Model file for the job. Use its own axes, mm. Face numbers are marked on the shaded views. A direction names the side the tool comes from. Round coordinates to 2 decimals unless told otherwise and drop trailing zeros. Loops run counter-clockwise (first coordinate to the right, second up) from the corner with the lowest first, then second, coordinate; pieces in that order, holes last. Notation, with made-up numbers: (64, 49.5) -> (106, 49.5) arc R27 cw to (106, 86.5) -> close; hole circle Ø7 at (34, -23). An arc over 180 degrees is marked (long way). Use a Markdown table: item, result.
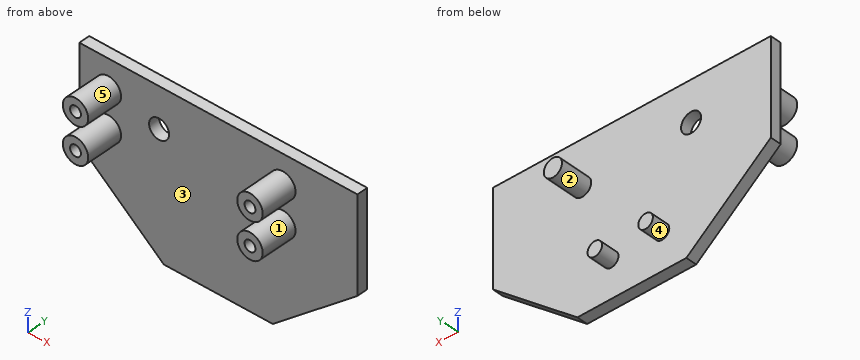
from build123d import *

# Parameters (mm, degrees)
SKETCH1_R             = 3.5
SKETCH1_R_2           = 1.5
BOSS_EXTRUDE1_DEPTH   = 10
BOSS_EXTRUDE1_2_DEPTH = 10
BOSS_EXTRUDE1_3_DEPTH = 10
BOSS_EXTRUDE1_4_DEPTH = 10
BOSS_EXTRUDE2_DEPTH   = 3
SKETCH3_R             = 2.75
CUT_EXTRUDE1_DEPTH    = 4
SKETCH4_R             = 2.5
BOSS_EXTRUDE3_DEPTH   = 8.9
SKETCH5_R             = 2
BOSS_EXTRUDE4_DEPTH   = 5


with BuildPart() as part:
    # Sketch1 → Boss-Extrude1 (new body)
    with BuildSketch(Plane(origin=(0, 0, 0), x_dir=(1, 0, 0), z_dir=(0, 1, 0))):
        with Locations(Location((0, 0, 0), (0, 0, 270))):
            Circle(SKETCH1_R)
        with Locations(Location((0, 0, 0), (0, 0, 270))):
            Circle(SKETCH1_R_2, mode=Mode.SUBTRACT)
    extrude(amount=BOSS_EXTRUDE1_DEPTH)



with BuildPart() as body_2:
    # Sketch1 → Boss-Extrude1 2 (new body)
    with BuildSketch(Plane(origin=(0, 0, 0), x_dir=(1, 0, 0), z_dir=(0, 1, 0))):
        with Locations(Location((0, -10, 0), (0, 0, 270))):
            Circle(SKETCH1_R)
        with Locations(Location((0, -10, 0), (0, 0, 270))):
            Circle(SKETCH1_R_2, mode=Mode.SUBTRACT)
    extrude(amount=BOSS_EXTRUDE1_2_DEPTH)


with BuildPart() as body_3:
    # Sketch1 → Boss-Extrude1 3 (new body)
    with BuildSketch(Plane(origin=(0, 0, 0), x_dir=(1, 0, 0), z_dir=(0, 1, 0))):
        with Locations(Location((48, -10, 0), (0, 0, 270))):
            Circle(SKETCH1_R)
        with Locations(Location((48, -10, 0), (0, 0, 270))):
            Circle(SKETCH1_R_2, mode=Mode.SUBTRACT)
    extrude(amount=BOSS_EXTRUDE1_3_DEPTH)


with BuildPart() as body_4:
    # Sketch1 → Boss-Extrude1 4 (new body)
    with BuildSketch(Plane(origin=(0, 0, 0), x_dir=(1, 0, 0), z_dir=(0, 1, 0))):
        with Locations(Location((48, 0, 0), (0, 0, 270))):
            Circle(SKETCH1_R)
        with Locations(Location((48, 0, 0), (0, 0, 270))):
            Circle(SKETCH1_R_2, mode=Mode.SUBTRACT)
    extrude(amount=BOSS_EXTRUDE1_4_DEPTH)


with BuildPart() as part_1:
    add(part.part)

    add(body_2.part)  # Boss-Extrude2 merges body 2

    add(body_3.part)  # Boss-Extrude2 merges body 3

    add(body_4.part)  # Boss-Extrude2 merges body 4
    # Sketch2 → Boss-Extrude2 (add)
    with BuildSketch(Plane(origin=(0, 10, 0), x_dir=(1, 0, 0), z_dir=(0, 1, 0))):
        Polygon((-8, -18), (-8, 8), (15.25, 27), (45.25, 27), (68.5, 8), (68.5, -18), align=None)
    extrude(amount=BOSS_EXTRUDE2_DEPTH)

    # Sketch3 → Cut-Extrude1 (cut)
    with BuildSketch(Plane.XZ.offset(-10)):
        with Locations(Location((13.95, 7, 0), (0, 0, 270))):
            Circle(SKETCH3_R)
    extrude(amount=-CUT_EXTRUDE1_DEPTH, mode=Mode.SUBTRACT)

    # Sketch4 → Boss-Extrude3 (add)
    with BuildSketch(Plane(origin=(0, 13, 0), x_dir=(1, 0, 0), z_dir=(0, 1, 0))):
        with Locations(Location((43.919609607, -5.65, 0), (0, 0, 90))):
            Circle(SKETCH4_R)
    extrude(amount=BOSS_EXTRUDE3_DEPTH)

    # Sketch5 → Boss-Extrude4 (add)
    with BuildSketch(Plane(origin=(0, 13, 0), x_dir=(1, 0, 0), z_dir=(0, 1, 0))):
        with Locations(Location((21.95, 17, 0), (0, 0, 90))):
            Circle(SKETCH5_R)
        with Locations(Location((35.919609607, 17, 0), (0, 0, 90))):
            Circle(SKETCH5_R)
    extrude(amount=BOSS_EXTRUDE4_DEPTH)


solid = part_1.part
Q1. Tool access for the marked faces 4 and 5: list every direction of +Z, -Z, +X, -X, +Y, -Y with a clear straight run to the whole face (end or side of a thin tool).
Results list:
| item | result |
|---|---|
| face 4 | +Y |
| face 5 | -Y |
Q2. Band-saw the part on A-A, the plane y = 5.5. Give the cut face in (x, z).
Results list:
| item | result |
|---|---|
| outline | circle Ø7 at (0, 0); circle Ø7 at (0, 10); circle Ø7 at (48, 0); circle Ø7 at (48, 10); hole circle Ø3 at (0, 0); hole circle Ø3 at (0, 10); hole circle Ø3 at (48, 0); hole circle Ø3 at (48, 10) |
Q3. Band-saw the part on C-C, the plane x = 13.95. Give the cut face in (y, z), plus the area to 3 significant figures.
Results list:
| item | result |
|---|---|
| outline | (10, -25.94) -> (13, -25.94) -> (13, 4.25) -> (10, 4.25) -> close; (10, 9.75) -> (13, 9.75) -> (13, 18) -> (10, 18) -> close |
| area | 115 mm² |
Q4. Flat gauge pins, fed straight in: pin 1 (2.5 mm diameter, centred on x = 0, z = 0, fed in from -Y); pin 2 (8 mm diameter, centred on x = 5.5, z = 1, fed in from +Y); pin 3 (1 mm diameter, centred on y = 11, z = -17.5, fed in from +X). Where does each tip first touch, or does it go through?
Results list:
| item | result |
|---|---|
| pin 1 | stops at y = 10 |
| pin 2 | stops at y = 13 |
| pin 3 | stops at x = 57.49 |
Q5. Pull direction X, two halves, no side cores. Call the marked faces 1, 2 and 3: released by +X, released by -X, zero draft, split by the parting line, or undercut.
Results list:
| item | result |
|---|---|
| face 1 | undercut |
| face 2 | split by the parting line |
| face 3 | undercut |
Q6. Drill centre lines: L1, parallel to X at y = 5.5, z = 0; L2, parallel to X at y = 17.75, z = -17; L3, parallel to Y at x = 8.5, z = 11. Where is each one in solid material? Low to high. Write a range as from..to.
Results list:
| item | result |
|---|---|
| L1 | x = -3.5..-1.5, 1.5..3.5, 44.5..46.5, 49.5..51.5 |
| L2 | x = 19.95..23.95, 33.92..37.92 |
| L3 | y = 10..13 |
Q7. Band-saw the part on B-B, the plane y = 11.25. Give the cut face in (x, z), plus the area to 3 significant figures.
Results list:
| item | result |
|---|---|
| outline | (-8, -8) -> (15.25, -27) -> (45.25, -27) -> (68.5, -8) -> (68.5, 18) -> (-8, 18) -> close; hole circle Ø5.5 at (13.95, 7) |
| area | 2,980 mm² |
Q8. Band-saw the part on D-D, the plane z = 5.65. Give the cut face in (x, y), plus the area to 3 significant figures.
Results list:
| item | result |
|---|---|
| outline | (-8, 10) -> (11.55, 10) -> (11.55, 13) -> (-8, 13) -> close; (16.35, 10) -> (68.5, 10) -> (68.5, 13) -> (46.42, 13) -> (46.42, 21.9) -> (41.42, 21.9) -> (41.42, 13) -> (16.35, 13) -> close |
| area | 260 mm² |
